Source: CAD feature listing. Evaluate the final solid. Frame: model axes, mm. A direction names the side the tool comes from. Coordinates: 2 decimals unless noted, no trailing zeros. Write each loop counter-clockwise with the first axis right and the second up, starting at its lowest first coordinate (ties: lowest second). Pieces come first, ordered by that corner, then holes. Notation, with made-up numbers: M 13.5,19 L 68.5,19 A28 ccw 68.5,54 Z; hole C 76.25,59 d1. An arc over 180 degrees is marked long. One line per item, written item: value. Start each with the question number.
Item 1: Ray query, L1, parallel to Y at x = 69, z = 0; L2, parallel to Z at x = 37, y = 14.5; L3, parallel to Z at x = 80, y = 4.25. Return the intervals inside material, ascending. Write a range as from..to.
Item 2: Cut plane B-B, the plane z = 0. Output: boundary loops of the cut face in (x, y), then the cut area to 3 significant figures.
Item 3: Pin query (flat end, axial travel): P1, Ø0.5, axis at x = 63, y = 14.5, coming from the +Z side; P2, Ø0.5, axis at x = 39, y = 14.5, coming from the -Z side. Return the tip coordinate at first contact, or that it passes through.
Item 4: Cut plane D-D, the plane z = -9. Output: boundary loops of the cut face in (x, y), then the cut area to 3 significant figures.
Item 5: Cut plane C-C, the plane y = 21.5. Output: boundary loops of the cut face in (x, z), then the cut area to 3 significant figures.
Item 6: Cut plane A-A, the plane x = 77. Output: boundary loops of the cut face in (y, z), then the cut area to 3 significant figures.
Item 7: Mould query, pull axis Z, two halves, no side actions, for faces 4 (the cylindrical face through (49.3, 20.244, 7.589)), 5 (the cylindrical face through (49.307, 24.227, 0.358)), 6 (the flat face through (49, 0, 0)). Classes: released by +Z, released by -Z, zero draft, split by the parting line, or undercut.
Item 8: Set-up query: faces 1 (the flat face through (49, 14, 6)), 2 (the cylindrical face through (49.3, 20.38, -7.68)), 3 (the cylindrical face through (49.307, 3.815, 0.596)). Return all of +Z, -Z, +X, -X, +Y, -Y with unobstructed straight access to the full face (end or side cutting, diameter ignored); none if empty.
```python
from build123d import *

# Parameters (mm, degrees)
SKETCH_1_R      = 2.75
EXTRUDE_1_DEPTH = 100
FILLET_1_R      = 10
CHAMFER_1_SIZE  = 0.5


with BuildPart() as part:
    # 草图1 → 凸台-拉伸1 (new body)
    with BuildSketch(Plane(origin=(0, 0, 0), x_dir=(0, 0, -1), z_dir=(1, 0, 0))):
        Polygon((-12, 0), (12, 0), (12, 4), (6, 4), (6, 24), (12, 24), (12, 28), (-12, 28), (-12, 24), (-6, 24), (-6, 4), (-12, 4), align=None)
        with Locations((0, 21.5)):
            Circle(SKETCH_1_R, mode=Mode.SUBTRACT)
        with Locations((0, 6.5)):
            Circle(SKETCH_1_R, mode=Mode.SUBTRACT)
    extrude(amount=EXTRUDE_1_DEPTH)

    # 圆角1
    # the kernel refuses this fillet: 10 mm, written as the material it adds along each edge
    with BuildSketch(Plane(origin=(0, 24, -6), x_dir=(0, -1, 0), z_dir=(1, 0, 0)), Plane(origin=(0, 4, 6), x_dir=(0, 1, 0), z_dir=(1, 0, 0))) as fillet_1_piece_1:
        with BuildLine():
            CenterArc((9.16515139, 10), FILLET_1_R, 203.578178478, 66.421821522)
            Line((0, 6), (-0.183303028, 5.92))
            ThreePointArc((-0.183303028, 5.92), (-0.2, 3), (-0.2, 0))
            Line((-0.2, 0), (0, -0.2))
            Line((0, -0.2), (9.16515139, -0.2))
            Line((9.16515139, -0.2), (9.16515139, 0))
        make_face()
    extrude(amount=100)
    with BuildSketch(Plane(origin=(0, 4, -6), x_dir=(0, 0, -1), z_dir=(1, 0, 0)), Plane(origin=(0, 24, 6), x_dir=(0, 0, 1), z_dir=(1, 0, 0))) as fillet_1_piece_2:
        with BuildLine():
            CenterArc((10, 9.16515139), FILLET_1_R, 180, 66.421821522)
            Line((0, 9.16515139), (-0.2, 9.16515139))
            Line((-0.2, 9.16515139), (-0.2, 0))
            Line((-0.2, 0), (0, -0.2))
            ThreePointArc((0, -0.2), (3, -0.2), (5.92, -0.183303028))
            Line((5.92, -0.183303028), (6, 0))
        make_face()
    extrude(amount=100)

    # 倒角1
    chamfer_1_edges = [part.edges().sort_by_distance(p)[0] for p in [
        (0, 21.5, 2.75),
        (100, 21.5, 2.75),
        (0, 6.5, 2.75),
        (100, 6.5, 2.75),
    ]]
    chamfer(chamfer_1_edges, length=CHAMFER_1_SIZE)


solid = part.part
```
From the geometry:
1. L1: y = 0..3.75, 9.25..18.75, 24.25..28
1. L2: z = -6..6
1. L3: z = -11.47..-1.58, 1.58..11.47
2. outline: M 0,0 L 100,0 L 100,3.25 L 99.5,3.75 L 0.5,3.75 L 0,3.25 Z; M 0,9.75 L 0.5,9.25 L 99.5,9.25 L 100,9.75 L 100,18.25 L 99.5,18.75 L 0.5,18.75 L 0,18.25 Z; M 0,24.75 L 0.5,24.25 L 99.5,24.25 L 100,24.75 L 100,28 L 0,28 Z
2. area: 1,700 mm²
3. P1: stops at z = 6
3. P2: stops at z = -6
4. outline: M 0,0 L 100,0 L 100,6.02 L 0,6.02 Z; M 0,21.98 L 100,21.98 L 100,28 L 0,28 Z
4. area: 1,200 mm²
5. outline: M 0,-8.55 L 100,-8.55 L 100,-3.25 L 99.5,-2.75 L 0.5,-2.75 L 0,-3.25 Z; M 0,3.25 L 0.5,2.75 L 99.5,2.75 L 100,3.25 L 100,8.55 L 0,8.55 Z
5. area: 1,160 mm²
6. outline: M 0,-12 L 4,-12 A10 cw 13.17,-6 L 14.83,-6 A10 cw 24,-12 L 28,-12 L 28,12 L 24,12 A10 cw 14.83,6 L 13.17,6 A10 cw 4,12 L 0,12 Z; hole C 6.5,0 d5.5; hole C 21.5,0 d5.5
6. area: 446 mm²
7. face 4: released by +Z
7. face 5: undercut
7. face 6: zero draft
8. face 1: +Z, +X, -X
8. face 2: -Z, +X, -X
8. face 3: +X, -X
